The drawing under review shows one solid part. Ordinate dimensions are in mm from its lowest x, y, z. A direction names the side the tool comes from. Coordinates: 2 decimals unless noted, no trailing zeros. Order: outer loops, then holes, each group sorted by start corner. A loop starts at its lowest first (then second) coordinate and runs counter-clockwise, first axis right, second up.
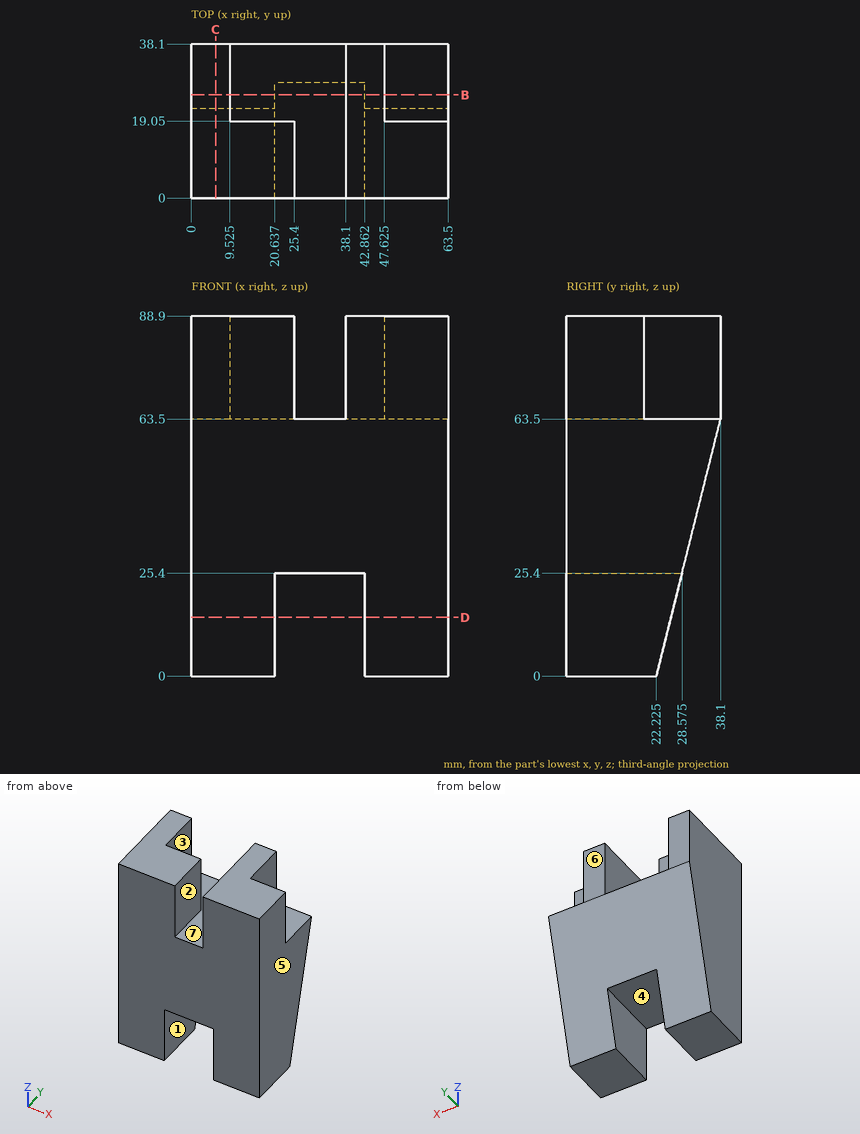
1. To check wall thickness, follow line 1 (X direction, y = 11, z = 64); line 2 (X direction, y = 3, z = 19); line 3 (Z direction, x = 23, y = 23.5). State the ranges of each line that lie inside material, in increasing order.
2. Add section B-B (y = 25.5). Give the boundary of the cut face in (x, z) (1 decimal).
3. Add section D-D (z = 14.5). Give the boundary of the cut face in (x, y).
4. For the marked faces 1, 2 and 3, list the 3-axis set-ups (+Z, -Z, +X, -X, +Y, -Y) from which the entire face can be reached by the end or side of a thin tool; tool diameter is ignored.
5. Insertion check: pin 1 (5 mm diameter, centred on x = 59.5, y = 29, fed in from +Z); pin 2 (4 mm diameter, centred on y = 33.5, z = 62.5, fed in from -X); pin 3 (5.5 mm diameter, centred on y = 30, z = 78.5, fed in from +X) (1 decimal); pin 4 (17.5 mm diameter, centred on x = 57.5, z = 79, fed in from +Y). Each pin has a flat end and moves straight along its axis. Give the tip position at first contact, or say it passes through.
6. Add section C-C (x = 6). Give the boundary of the cut face in (y, z) (1 decimal).
7. Mouldability with a two-part tool opening along X and no side actions: class the marked faces 4, 5, 6 and 7 as pulls with the +X half, pulls with the -X half, needs draft (parallel to the pull), parting line crosses it, or undercut.
Solution:
1. line 1: x = 0 to 25.4, 38.1 to 63.5
1. line 2: x = 0 to 20.64, 42.86 to 63.5
1. line 3: z = 25.4 to 63.5
2. outline: (0, 13.1) - (20.6, 13.1) - (20.6, 25.4) - (42.9, 25.4) - (42.9, 13.1) - (63.5, 13.1) - (63.5, 63.5) - (47.6, 63.5) - (47.6, 88.9) - (38.1, 88.9) - (38.1, 63.5) - (9.5, 63.5) - (9.5, 88.9) - (0, 88.9) - close
3. outline: (0, 0) - (20.64, 0) - (20.64, 25.85) - (0, 25.85) - close; (42.86, 0) - (63.5, 0) - (63.5, 25.85) - (42.86, 25.85) - close
4. face 1: -Z, +Y, -Y
4. face 2: +Z, +Y, -Y
4. face 3: +Z, +Y
5. pin 1: stops at z = 63.5
5. pin 2: stops at x = 0
5. pin 3: stops at x = 47.6
5. pin 4: stops at y = 19.05
6. outline: (0, 0) - (22.2, 0) - (38.1, 63.5) - (38.1, 88.9) - (0, 88.9) - close
7. face 4: undercut
7. face 5: pulls with the +X half
7. face 6: needs draft
7. face 7: undercut
